```python
from build123d import *

# Parameters (mm, degrees)
STRUCTURAL_MEMBER1_DEPTH = 330.2
SKETCH15_R               = 6.35
CUT_EXTRUDE1_DEPTH       = 229.688177438
SKETCH16_R               = 12.7
CUT_EXTRUDE2_DEPTH       = 229.688177438
LPATTERN1_COUNT          = 4
LPATTERN1_PITCH          = 38.1


with BuildPart() as part:
    # Sketch13 → Structural Member1 (new body)
    with BuildSketch(Plane.ZY.offset(-107.95)):
        with BuildLine():
            Line((-14.2875, -38.1), (14.2875, -38.1))
            ThreePointArc((14.2875, -38.1), (17.655096045, -36.705096045), (19.05, -33.3375))
            Line((19.05, -33.3375), (19.05, 33.3375))
            ThreePointArc((19.05, 33.3375), (17.655096045, 36.705096045), (14.2875, 38.1))
            Line((14.2875, 38.1), (-14.2875, 38.1))
            ThreePointArc((-14.2875, 38.1), (-17.655096045, 36.705096045), (-19.05, 33.3375))
            Line((-19.05, 33.3375), (-19.05, -33.3375))
            ThreePointArc((-19.05, -33.3375), (-17.655096045, -36.705096045), (-14.2875, -38.1))
        make_face()
        with BuildLine():
            Line((-14.2875, -35.98418), (14.2875, -35.98418))
            ThreePointArc((14.2875, -35.98418), (16.158985376, -35.208985376), (16.93418, -33.3375))
            Line((16.93418, -33.3375), (16.93418, 33.3375))
            ThreePointArc((16.93418, 33.3375), (16.158985376, 35.208985376), (14.2875, 35.98418))
            Line((14.2875, 35.98418), (-14.2875, 35.98418))
            ThreePointArc((-14.2875, 35.98418), (-16.158985376, 35.208985376), (-16.93418, 33.3375))
            Line((-16.93418, 33.3375), (-16.93418, -33.3375))
            ThreePointArc((-16.93418, -33.3375), (-16.158985376, -35.208985376), (-14.2875, -35.98418))
        make_face(mode=Mode.SUBTRACT)
    extrude(amount=STRUCTURAL_MEMBER1_DEPTH)

    # Sketch15 → Cut-Extrude1 (cut, through all)
    with BuildSketch(Plane(origin=(0, 0, -19.05), x_dir=(-1, 0, 0), z_dir=(0, 0, -1))):
        with Locations(Location((-95.25, 0, 0), (0, 0, 90))):
            Circle(SKETCH15_R)
        with Locations(Location((209.55, 0, 0), (0, 0, 90))):
            Circle(SKETCH15_R)
    extrude(amount=-CUT_EXTRUDE1_DEPTH, mode=Mode.SUBTRACT)

    # Sketch16 → Cut-Extrude2 (cut, through all)
    with BuildSketch(Plane(origin=(0, 0, -19.05), x_dir=(-1, 0, 0), z_dir=(0, 0, -1))):
        with Locations(Location((22.225, 16.497783942, 0), (0, 0, 90))):
            Circle(SKETCH16_R)
        with Locations(Location((41.275, -16.497783942, 0), (0, 0, 90))):
            Circle(SKETCH16_R)
    cut_extrude2 = extrude(amount=-CUT_EXTRUDE2_DEPTH, mode=Mode.SUBTRACT)

    # LPattern1: Cut-Extrude2 ×4
    with Locations(*[(-i * LPATTERN1_PITCH, 0, 0) for i in range(1, LPATTERN1_COUNT)]):
        add(cut_extrude2, mode=Mode.SUBTRACT)


solid = part.part
```
Could you check a few things on this model? Use its own coordinates, in mm. A direction names the side the tool comes from. Round coordinates to 2 decimals unless told otherwise and drop trailing zeros. Loops run counter-clockwise (first coordinate to the right, second up) from the corner with the lowest first, then second, coordinate; pieces in that order, holes last. Notation, with made-up numbers: (75, 62) - (110, 62) arc R8 cw to (110, 73) - close; hole circle Ø1 at (69, -24.5). An arc over 180 degrees is marked (long way). Answer in a Markdown table with one row per item. Add a question column.
(1) If we section it at C-C (y = 0): Please give me the cut outline in (x, z), plus the area to 3 significant figures.
(2) If we section it at B-B (z = 8): Please give me the cut outline in (x, y).
(3) For faces 4 (the face through (-55, 38.1, 0)), 5 (the face through (-55, 35.984, 0)), which set-ups out of +Z, -Z, +X, -X, +Y, -Y let a thin tool reach every point of the face, with its end or its side?
(4) If we mould it in two halves opening along Z, with no side actions, what happens to faces 1 (the face through (-123.933, 14.844, -18.007)), 2 (the face through (-55, 0, -19.05)), 3 (the face through (-55, 0, 16.934))? For each: pulls with the +Z half, pulls with the -Z half, needs draft (parallel to the pull), parting line crosses it, or undercut.
(5) I need wall thicknesses on line 1 along Y through (x, z) = (-53.5, 7); line 2 along X through (y, z) = (0, 17.9); line 3 along Z through (x, y) = (-197, -17). Which ranges of each line are inside material? Lowest first, please.
Model answer:
| question | item | result |
|---|---|---|
| 1 | outline | (-222.25, -19.05) - (-215.9, -19.05) - (-215.9, -16.93) - (-222.25, -16.93) - close; (-222.25, 16.93) - (-215.9, 16.93) - (-215.9, 19.05) - (-222.25, 19.05) - close; (-203.2, -19.05) - (88.9, -19.05) - (88.9, -16.93) - (-203.2, -16.93) - close; (-203.2, 16.93) - (88.9, 16.93) - (88.9, 19.05) - (-203.2, 19.05) - close; (101.6, -19.05) - (107.95, -19.05) - (107.95, -16.93) - (101.6, -16.93) - close; (101.6, 16.93) - (107.95, 16.93) - (107.95, 19.05) - (101.6, 19.05) - close |
| 1 | area | 1,290 mm² |
| 2 | outline | (-222.25, -38.1) - (107.95, -38.1) - (107.95, -35.98) - (-222.25, -35.98) - close; (-222.25, 35.98) - (107.95, 35.98) - (107.95, 38.1) - (-222.25, 38.1) - close |
| 3 | face 4 | +Z, -Z, +X, -X, +Y |
| 3 | face 5 | +X, -X |
| 4 | face 1 | needs draft |
| 4 | face 2 | pulls with the -Z half |
| 4 | face 3 | undercut |
| 5 | line 1 | y = -38.1 to -35.98, 35.98 to 38.1 |
| 5 | line 2 | x = -222.25 to -215.9, -203.2 to 88.9, 101.6 to 107.95 |
| 5 | line 3 | z = -19.05 to -16.93, 16.93 to 19.05 |
